Job drawing, mm, ordinate dimensions from the low corner. One solid piece. A direction names the side the tool comes from. Round coordinates to 2 decimals unless told otherwise and drop trailing zeros. Loops run counter-clockwise (first coordinate to the right, second up) from the corner with the lowest first, then second, coordinate; pieces in that order, holes last.
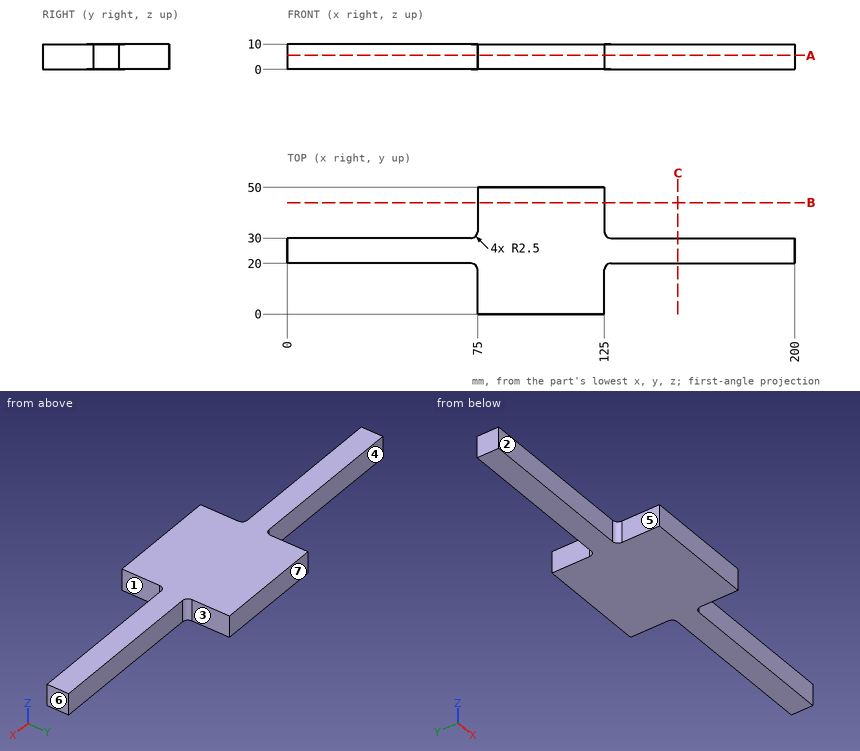
1) Slice it at A-A, the plane z = 5.5. Give the cut face in (x, y), then the cut area to 3 significant figures.
Values:
outline: (0, 20) - (72.5, 20) arc R2.5 cw to (75, 17.5) - (75, 0) - (125, 0) - (125, 17.5) arc R2.5 cw to (127.5, 20) - (200, 20) - (200, 30) - (127.5, 30) arc R2.5 cw to (125, 32.5) - (125, 50) - (75, 50) - (75, 32.5) arc R2.5 cw to (72.5, 30) - (0, 30) - close
area: 4,010 mm2
2) Mould opens along X. For the marked faces 5, 6 and 7 say: released by +X, released by -X, zero draft, split by the parting line, or undercut.
Values:
face 5: released by -X
face 6: released by +X
face 7: zero draft
3) Tool access for the marked faces 1, 2, 3 and 4: list every direction of +Z, -Z, +X, -X, +Y, -Y with a clear straight run to the whole face (end or side of a thin tool).
Values:
face 1: +Z, -Z, +X, -Y
face 2: +Z, -Z, -X, -Y
face 3: +Z, -Z, +X, +Y
face 4: +Z, -Z, -X, +Y
4) Slice it at C-C, the plane x = 154. Give the cut face in (y, z).
Values:
outline: (20, 0) - (30, 0) - (30, 10) - (20, 10) - close
5) Wall check: line 1 along X through (y, z) = (45, 3.75); line 2 along Y through (x, z) = (168, 4.5); line 3 along Y through (x, z) = (126, 7.75). Give the ranges that are in metal, low to high.
Values:
line 1: x = 75 to 125
line 2: y = 20 to 30
line 3: y = 19.5 to 30.5
6) Drop flat-ended pins along their axis: pin 1 Ø6 at (y, z) = (19, 2.5) entering from -X; pin 2 Ø2 at (y, z) = (37, 6) entering from +X; pin 3 Ø3 at (x, z) = (47, 7.5) entering from +Y; pin 4 Ø5 at (y, z) = (39, 5.5) entering from -X. Give the stop position or say it passes through.
Values:
pin 1: stops at x = 0
pin 2: stops at x = 125
pin 3: stops at y = 30
pin 4: stops at x = 75
7) Slice it at B-B, the plane y = 44. Give the cut face in (x, z), then the cut area to 3 significant figures.
Values:
outline: (75, 0) - (125, 0) - (125, 10) - (75, 10) - close
area: 500 mm2
